Verification items for the finished model (mm, model axes). Face numbers are marked on the shaded views. A direction names the side the tool comes from. Round coordinates to 2 decimals unless told otherwise and drop trailing zeros. Write each loop counter-clockwise with the first axis right and the second up, starting at its lowest first coordinate (ties: lowest second). Pieces come first, ordered by that corner, then holes. Notation, with made-up numbers: (-27.5, 54) - (-16.5, 54) arc R20 cw to (-16.5, 92) - close; hole circle Ø5 at (80.25, -20). An arc over 180 degrees is marked (long way). Answer as a JSON object with one key per item and string values.
```python
from build123d import *

# Parameters (mm, degrees)
SALIENTE_EXTRUIR1_DEPTH      = 12
SALIENTE_EXTRUIR2_DEPTH      = 10
SALIENTE_EXTRUIR2_DEPTH_BACK = 12
CROQUIS3_R                   = 1.1
CORTAR_EXTRUIR1_DEPTH        = 4.912531407
REDONDEO1_R                  = 0.5


with BuildPart() as part:
    # Croquis1 → Saliente-Extruir1 (new body)
    with BuildSketch(Plane(origin=(0, 0, 0), x_dir=(0, 0, -1), z_dir=(1, 0, 0))):
        with BuildLine():
            Line((-2.1, 3.987468593), (2.1, 3.987468593))
            ThreePointArc((2.1, 3.987468593), (0, -4.506651282), (-2.1, 3.987468593))
        make_face()
        with BuildLine():
            Line((-1.85, 2.487468593), (1.85, 2.487468593))
            ThreePointArc((1.85, 2.487468593), (0, -3.1), (-1.85, 2.487468593))
        make_face(mode=Mode.SUBTRACT)
    extrude(amount=SALIENTE_EXTRUIR1_DEPTH)

    # Croquis2 → Saliente-Extruir2 (add, two sides: drawn at the far end of the back side and taken through both)
    with BuildSketch(Plane(origin=(12, 0, 0), x_dir=(0, 0, -1), z_dir=(1, 0, 0)).offset(-SALIENTE_EXTRUIR2_DEPTH_BACK)):
        Polygon((-4.272391992, -7.4), (4.272391992, -7.4), (8.544783984, 0), (4.272391992, 7.4), (-4.272391992, 7.4), (-8.544783984, 0), align=None)
        with BuildLine():
            Line((-1.85, 2.487468593), (1.85, 2.487468593))
            ThreePointArc((1.85, 2.487468593), (0, -3.1), (-1.85, 2.487468593))
        make_face(mode=Mode.SUBTRACT)
    extrude(amount=SALIENTE_EXTRUIR2_DEPTH + SALIENTE_EXTRUIR2_DEPTH_BACK)

    # Croquis3 → Cortar-Extruir1 (cut)
    with BuildSketch(Plane.XZ.offset(-2.487468593)):
        with Locations(Location((7.375, 0, 0), (0, 0, 270))):
            Circle(CROQUIS3_R)
    extrude(amount=-CORTAR_EXTRUIR1_DEPTH, mode=Mode.SUBTRACT)

    # Redondeo1
    redondeo1_edges = [part.edges().sort_by_distance(p)[0] for p in [
        (0, 2.487468593, 0),
        (22, -3.7, 6.408587988),
        (22, -7.4, 0),
        (22, -3.7, -6.408587988),
        (22, 3.7, -6.408587988),
        (22, 7.4, 0),
        (22, 3.7, 6.408587988),
        (0, -3.7, 6.408587988),
        (0, -7.4, 0),
        (0, -3.7, -6.408587988),
        (0, 3.7, -6.408587988),
        (0, 7.4, 0),
        (0, 3.7, 6.408587988),
        (22, -3.1, 0),
        (22, 2.487468593, 0),
        (0, -3.1, 0),
    ]]
    fillet(redondeo1_edges, radius=REDONDEO1_R)


solid = part.part
```
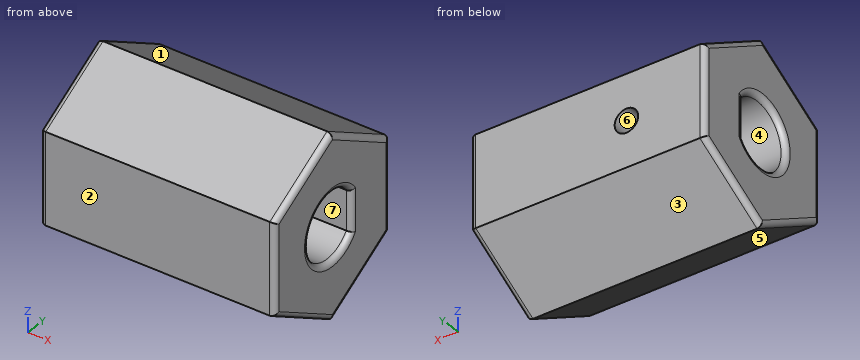
Q1. Gauge pin test, flat ends, axial feed: P1, Ø1, axis at x = 6, y = -3.5, coming from the -Z side; P2, Ø1.5, axis at x = 10, z = -6, coming from the +Y side; P3, Ø1.5, axis at y = -2, z = 0.5, coming from the -X side; P4, Ø1, axis at x = 10, y = 5, coming from the +Z side. Record the tip position at first contact, or that the pin passes through.
Geometry check:
{"P1": "stops at z = -6.81", "P2": "stops at y = 5.71", "P3": "passes through", "P4": "stops at z = 5.95"}
Q2. Section check A-A, the plane z = 0. Record the cut outline in (x, y) (3 decimals), then the cut area to 3 significant figures.
Geometry check:
{"outline": "(0, -6.9) arc R0.5 ccw to (0.5, -7.4) - (21.5, -7.4) arc R0.5 ccw to (22, -6.9) - (22, -3.6) arc R0.5 ccw to (21.5, -3.1) - (0.5, -3.1) arc R0.5 ccw to (0, -3.6) - close; (0, 2.987) arc R0.5 ccw to (0.5, 2.487) - (6.275, 2.487) - (6.275, 7.4) - (0.5, 7.4) arc R0.5 ccw to (0, 6.9) - close; (8.475, 2.487) - (21.5, 2.487) arc R0.5 ccw to (22, 2.987) - (22, 6.9) arc R0.5 ccw to (21.5, 7.4) - (8.475, 7.4) - close", "area": "191 mm2"}
Q3. Section check B-B, the plane x = 20. Record the cut outline in (y, z).
Geometry check:
{"outline": "(-7.4, -4.27) - (0, -8.54) - (7.4, -4.27) - (7.4, 4.27) - (0, 8.54) - (-7.4, 4.27) - close; hole (2.49, -1.85) - (2.49, 1.85) arc R3.1 ccw (long way) to start"}
Q4. Set-up check for the marked faces 5, 6 and 7: record each of +Z, -Z, +X, -X, +Y, -Y from which the full face is reachable in a straight line by a thin tool's end or side.
Geometry check:
{"face 5": "-Z, +X, -X, -Y", "face 6": "+Y", "face 7": "+X, -X"}
Q5. Release check for a two-part mould opening along Z. For the marked faces 1, 2, 3 and 4 record: released by +Z, released by -Z, zero draft, split by the parting line, or undercut.
Geometry check:
{"face 1": "released by +Z", "face 2": "zero draft", "face 3": "released by -Z", "face 4": "undercut"}
Q6. Material ranges on line 1 along X through (y, z) = (3.6, 0) (3 decimals); line 2 along Y through (x, z) = (14.75, 0); line 3 along Y through (x, z) = (2.5, -0.75), recorded low to high. Write a range as [from, to].
Geometry check:
{"line 1": "x = [0, 6.275], [8.475, 22]", "line 2": "y = [-7.4, -3.1], [2.49, 7.4]", "line 3": "y = [-7.4, -3.01], [2.49, 7.4]"}
